CAD build for the part. Positions are in the model's coordinates, mm. A direction names the side the tool comes from. Round coordinates to 2 decimals unless told otherwise and drop trailing zeros. Order: outer loops, then holes, each group sorted by start corner. A loop starts at its lowest first (then second) coordinate and runs counter-clockwise, first axis right, second up. Notation, with made-up numbers: M 50.5,-7 L 70.5,-7 A22 ccw 70.5,30 Z; hole C 77.25,-38.75 d2. An arc over 180 degrees is marked long. Answer as a JSON object with one key per item and string values.
```python
from build123d import *

# Parameters (mm, degrees)
F0_W      = 58.7
F0_H      = 124
F1_DEPTH  = 7.75
F5_R      = 8.15
F4_R      = 2.374986
F7_DEPTH  = 13
F8_DEPTH  = 0.9
F3_R      = 2.275
F3_W      = 5.8
F3_H      = 1.35
F9_DEPTH  = 0.9
F10_DEPTH = 0.9
F4_W      = 9
F4_H      = 3
F11_DEPTH = 12
F2_R      = 5.4
F12_DEPTH = 0.25
F14_DEPTH = 0.55
F15_SIZE  = 0.5
F2_W      = 51.7
F2_H      = 92
F16_DEPTH = 0.25


with BuildPart() as f1:
    # F0 (on Top) → F1 (new body)
    with BuildSketch(Plane.XY):
        with Locations((59.907148, 62)):
            Rectangle(F0_W, F0_H)
    extrude(amount=F1_DEPTH)

    # F5
    f5_edges = [f1.edges().sort_by_distance(p)[0] for p in [
        (30.557148, 124, 3.875),
        (89.257148, 124, 3.875),
        (30.557148, 0, 3.875),
        (89.257148, 0, 3.875),
    ]]
    fillet(f5_edges, radius=F5_R)

    # F4 (on face) → F7 (cut)
    with BuildSketch(Plane.XZ):
        with Locations((41.832148, 3.875)):
            Circle(F4_R)
    extrude(amount=-F7_DEPTH, mode=Mode.SUBTRACT)

    # F6 (on face) → F8 (join)
    with BuildSketch(Plane(origin=(0, 124, 0), x_dir=(-1, 0, 0), z_dir=(0, 1, 0))):
        with BuildLine():
            Line((-70.657148, 4.975), (-78.507148, 4.975))
            ThreePointArc((-78.507148, 4.975), (-79.607148, 3.875), (-78.507148, 2.775))
            Line((-78.507148, 2.775), (-70.657148, 2.775))
            ThreePointArc((-70.657148, 2.775), (-69.557148, 3.875), (-70.657148, 4.975))
        make_face()
    extrude(amount=F8_DEPTH)

    # F3 (on face) → F9 (join)
    with BuildSketch(Plane(origin=(30.557148, 0, 0), x_dir=(0, -1, 0), z_dir=(-1, 0, 0))):
        with Locations((-93.525, 3.875)):
            Circle(F3_R)
        with BuildLine():
            ThreePointArc((-80.7, 3.875), (-82.975, 6.15), (-85.25, 3.875))
            ThreePointArc((-85.25, 3.875), (-82.975, 1.6), (-80.7, 3.875))
        make_face()
        with Locations((-104.8, 4.55)):
            Rectangle(F3_W, F3_H)
    extrude(amount=F9_DEPTH)

    # F3 (on face) → F10 (cut)
    with BuildSketch(Plane(origin=(30.557148, 0, 0), x_dir=(0, -1, 0), z_dir=(-1, 0, 0))):
        with Locations((-104.8, 3.2)):
            Rectangle(F3_W, F3_H)
    extrude(amount=-F10_DEPTH, mode=Mode.SUBTRACT)

    # F4 (on face) → F11 (cut)
    with BuildSketch(Plane.XZ):
        with Locations((60.307148, 3.889738)):
            Rectangle(F4_W, F4_H)
    extrude(amount=-F11_DEPTH, mode=Mode.SUBTRACT)

    # F2 (on face) → F12 (cut)
    with BuildSketch(Plane.XY.offset(7.75)):
        with Locations((59.907148, 8.25)):
            Circle(F2_R)
    extrude(amount=-F12_DEPTH, mode=Mode.SUBTRACT)

    # F13 (on face) → F14 (cut)
    with BuildSketch(Plane.XY.offset(7.75)):
        with BuildLine():
            Line((38.707148, 0), (81.107148, 0))
            ThreePointArc((81.107148, 0), (86.870068, 2.38708), (89.257148, 8.15))
            Line((89.257148, 8.15), (89.257148, 115.85))
            ThreePointArc((89.257148, 115.85), (86.870068, 121.61292), (81.107148, 124))
            Line((81.107148, 124), (38.707148, 124))
            ThreePointArc((38.707148, 124), (32.944228, 121.61292), (30.557148, 115.85))
            Line((30.557148, 115.85), (30.557148, 8.15))
            ThreePointArc((30.557148, 8.15), (32.944228, 2.38708), (38.707148, 0))
        make_face()
        with BuildLine():
            Line((88.207148, 115.85), (88.207148, 8.15))
            ThreePointArc((88.207148, 8.15), (86.127606, 3.129542), (81.107148, 1.05))
            Line((81.107148, 1.05), (38.707148, 1.05))
            ThreePointArc((38.707148, 1.05), (33.68669, 3.129542), (31.607148, 8.15))
            Line((31.607148, 8.15), (31.607148, 115.85))
            ThreePointArc((31.607148, 115.85), (33.68669, 120.870458), (38.707148, 122.95))
            Line((38.707148, 122.95), (81.107148, 122.95))
            ThreePointArc((81.107148, 122.95), (86.127606, 120.870458), (88.207148, 115.85))
        make_face(mode=Mode.SUBTRACT)
    extrude(amount=-F14_DEPTH, mode=Mode.SUBTRACT)

    # F15
    f15_edges = [f1.edges().sort_by_distance(p)[0] for p in [
        (59.907148, 124, 7.2),
        (86.870068, 121.61292, 7.2),
        (89.257148, 62, 7.2),
        (86.870068, 2.38708, 7.2),
        (59.907148, 0, 7.2),
        (32.944228, 2.38708, 7.2),
        (30.557148, 62, 7.2),
        (32.944228, 121.61292, 7.2),
        (89.257148, 62, 0),
    ]]
    chamfer(f15_edges, length=F15_SIZE)

    # F2 (on face) → F16 (cut)
    with BuildSketch(Plane.XY.offset(7.75)):
        with Locations((59.907148, 62)):
            Rectangle(F2_W, F2_H)
    extrude(amount=-F16_DEPTH, mode=Mode.SUBTRACT)


solid = f1.part
```
Item 1: Wall check: line 1 along Y through (x, z) = (62.5, 7.25); line 2 along Y through (x, z) = (57, 5.5); line 3 along X through (y, z) = (111, 2.25). Give the ranges that are in metal, low to high. Write a range as [from, to].
Worked answers:
{"line 1": "y = [1.05, 122.95]", "line 2": "y = [0, 124]", "line 3": "x = [30.56, 89.26]"}
Item 2: Two-plate mould, pull along Y, no slides. Class faces 1 (the flat face through (60, 63, 7.5)), 2 (the flat face through (60, 12, 4)), 3 (the conical face through (86.677, 121.299, 0.142)): released by +Y, released by -Y, zero draft, split by the parting line, or undercut.
Worked answers:
{"face 1": "undercut", "face 2": "released by -Y", "face 3": "released by +Y"}
Item 3: Saw through at B-B on x = 58. List the corners of the cut face in (y, z), and give its area (3 significant figures).
Worked answers:
{"outline": "M 0,0.5 L 0.5,0 L 123.5,0 L 124,0.5 L 124,6.7 L 123.5,7.2 L 122.95,7.2 L 122.95,7.75 L 108,7.75 L 108,7.5 L 16,7.5 L 16,7.75 L 13.3,7.75 L 13.3,7.5 L 3.2,7.5 L 3.2,7.75 L 1.05,7.75 L 1.05,7.2 L 0.5,7.2 L 0,6.7 L 0,5.39 L 12,5.39 L 12,2.39 L 0,2.39 Z", "area": "898 mm2"}
Item 4: 3-axis set-ups, long thin cutter, end or side, ignore diameter. For faces 4 (the cylindrical face through (86.1, 120.9, 7.5)), 5 (the flat face through (60, 6, 5.39)), 6 (the flat face through (60, 8, 7.5)): which of +Z, -Z, +X, -X, +Y, -Y reach the whole face in a straight line?
Worked answers:
{"face 4": "+Z, +X, +Y", "face 5": "-Y", "face 6": "+Z"}
Item 5: Drop flat-ended pins along their axis: pin 1 Ø3 at (y, z) = (88.5, 7) entering from +X; pin 2 Ø0.7 at (x, z) = (31, 3.5) entering from -Y; pin 3 Ø1 at (x, z) = (30, 4.5) entering from +Y; pin 4 Ø4 at (x, z) = (56.5, 5.5) entering from +Y. Give the stop position or say it passes through.
Worked answers:
{"pin 1": "stops at x = 89.26", "pin 2": "stops at y = 4.64", "pin 3": "stops at y = 107.7", "pin 4": "stops at y = 124"}
Item 6: Saw through at A-A on y = 68.5. List the corners of the cut face in (x, z), and give its area (3 significant figures).
Worked answers:
{"outline": "M 30.56,0.5 L 31.06,0 L 88.76,0 L 89.26,0.5 L 89.26,6.7 L 88.76,7.2 L 88.21,7.2 L 88.21,7.75 L 85.76,7.75 L 85.76,7.5 L 34.06,7.5 L 34.06,7.75 L 31.61,7.75 L 31.61,7.2 L 31.06,7.2 L 30.56,6.7 Z", "area": "440 mm2"}
Item 7: Saw through at C-C on x = 75. List the corners of the cut face in (y, z) (3 decimals).
Worked answers:
{"outline": "M 0,0.5 L 0.5,0 L 123.5,0 L 124,0.5 L 124,2.775 L 124.9,2.775 L 124.9,4.975 L 124,4.975 L 124,6.7 L 123.5,7.2 L 122.95,7.2 L 122.95,7.75 L 108,7.75 L 108,7.5 L 16,7.5 L 16,7.75 L 1.05,7.75 L 1.05,7.2 L 0.5,7.2 L 0,6.7 Z"}
